Geometry check sheet. Reference: the model listing, model coordinates, mm. A direction names the side the tool comes from. Coordinates: 2 decimals unless noted, no trailing zeros. Write each loop counter-clockwise with the first axis right and the second up, starting at its lowest first coordinate (ties: lowest second). Pieces come first, ordered by that corner, then holes. Notation, with made-up numbers: (54, 32.25) - (67, 32.25) arc R12 cw to (67, 37.25) - close; hole circle Ø8 at (8, -0.75). An arc over 180 degrees is marked (long way). Answer as a JSON object with one key per item and string values. Group by question number.
from build123d import *

# Parameters (mm, degrees)
F5_DEPTH = 1.501
F6_R     = 1.25
F7_DEPTH = 0.8


with BuildPart() as f1:
    # F0 (on Front) → F1 (revolve)
    with BuildSketch(Plane.XZ):
        Polygon((0, 8), (0, 0), (2.3, 0), (2.3, 5), (1.5, 5), (1.5, 8), align=None)
    revolve(axis=Axis((1.15, 0, 0), (1, 0, 0)))

    # F2 (on Front) → F3 (revolve, cut)
    with BuildSketch(Plane.XZ):
        Polygon((0, 2.45), (0, 0), (2.3, 0), (2.3, 1.5), (0.9, 1.5), (0.9, 2.45), align=None)
    revolve(axis=Axis((1.15, 0, 0), (-1, 0, 0)), mode=Mode.SUBTRACT)

    # F4 (on face) → F5 (cut, through all)
    with BuildSketch(Plane.YZ.offset(1.5)):
        with BuildLine():
            ThreePointArc((7.35, 0), (6.5, 0.85), (5.65, 0))
            ThreePointArc((5.65, 0), (6.5, -0.85), (7.35, 0))
        make_face()
        with BuildLine():
            ThreePointArc((-2.4, -5.629165), (-2.513878, -5.204165), (-2.825, -4.893044))
            ThreePointArc((-2.825, -4.893044), (-3.986122, -6.054165), (-2.4, -5.629165))
        make_face()
        with BuildLine():
            ThreePointArc((-2.4, 5.629165), (-3.986122, 6.054165), (-2.825, 4.893044))
            ThreePointArc((-2.825, 4.893044), (-2.513878, 5.204165), (-2.4, 5.629165))
        make_face()
    extrude(amount=-F5_DEPTH, mode=Mode.SUBTRACT)

    # F6 (on face) → F7 (cut, through all)
    with BuildSketch(Plane.YZ.offset(2.3)):
        with Locations((-5, 0)):
            Circle(F6_R)
    extrude(amount=-F7_DEPTH, mode=Mode.SUBTRACT)


solid = f1.part
(1) Gauge pin test, flat end, axial feed: pin 1 (5.5 mm diameter, centred on y = 0, z = 0.5, fed in from -X). Record the tip position at first contact, or that the pin passes through.
(2) Section check C-C (z = 0.5). Record the cut outline in (x, y).
(3) Material ranges on L1, parallel to Y at x = 0.5, z = 0; L2, parallel to Y at x = 1.1, z = 0; L3, parallel to Z at x = 0.1, y = -3.5, recorded low to high. Write a range as [from, to].
(4) Set-up check for faces 1 (the face through (1.5, 5.2, 0.1)), 2 (the face through (1.91, -3.75, -0.03)), 3 (the face through (0.74, 7.81, -1.73)), 4 (the face through (0.9, -2, 0)), 5 (the face through (2.3, 2, 0)): record each of +Z, -Z, +X, -X, +Y, -Y from which the full face is reachable in a straight line by a thin tool's end or side.
(5) Section check B-B (y = 0). Record the cut outline in (x, z).
(6) Section check A-A (x = 0.7). Record the cut outline in (y, z) (3 decimals).
(7) Section check D-D (y = -3.25). Record the cut outline in (x, z).
Conclusion:
{
 "1": {"pin 1": "stops at x = 0"},
 "2": {"outline": "(0, -7.98) - (1.5, -7.98) - (1.5, -3.85) - (2.3, -3.85) - (2.3, -1.41) - (0.9, -1.41) - (0.9, -2.4) - (0, -2.4) - close; (0, 2.4) - (0.9, 2.4) - (0.9, 1.41) - (2.3, 1.41) - (2.3, 4.97) - (1.5, 4.97) - (1.5, 5.81) - (0, 5.81) - close; (0, 7.19) - (1.5, 7.19) - (1.5, 7.98) - (0, 7.98) - close"},
 "3": {"L1": "y = [-8, -2.45], [2.45, 5.65], [7.35, 8]", "L2": "y = [-8, -1.5], [1.5, 5.65], [7.35, 8]", "L3": "z = [-7.19, -6.44], [-4.82, 4.82], [6.44, 7.19]"},
 "4": {"face 1": "+X", "face 2": "+X, -Y", "face 3": "+X, -X", "face 4": "-X", "face 5": "+Z, -Z, +X, +Y, -Y"},
 "5": {"outline": "(0, -8) - (1.5, -8) - (1.5, -5) - (2.3, -5) - (2.3, -1.5) - (0.9, -1.5) - (0.9, -2.45) - (0, -2.45) - close; (0, 2.45) - (0.9, 2.45) - (0.9, 1.5) - (2.3, 1.5) - (2.3, 5) - (1.5, 5) - (1.5, 8) - (0, 8) - close"},
 "6": {"outline": "circle Ø16 at (0, 0); hole (-2.825, -4.893) arc R0.85 ccw (long way) to (-2.4, -5.629) arc R0.85 ccw to start; hole (-2.825, 4.893) arc R0.85 ccw to (-2.4, 5.629) arc R0.85 ccw (long way) to start; hole circle Ø4.9 at (0, 0); hole circle Ø1.7 at (6.5, 0)"},
 "7": {"outline": "(0, -7.31) - (1.5, -7.31) - (1.5, -6.48) - (0, -6.48) - close; (0, -4.78) - (1.5, -4.78) - (1.5, -3.8) - (2.3, -3.8) - (2.3, 3.8) - (1.5, 3.8) - (1.5, 4.78) - (0, 4.78) - close; (0, 6.48) - (1.5, 6.48) - (1.5, 7.31) - (0, 7.31) - close"}
}
